Check sheet for the modelled part. Datum: model origin and axes. Units: mm. A direction names the side the tool comes from. Coordinates: 2 decimals unless noted, no trailing zeros. Order: outer loops, then holes, each group sorted by start corner. A loop starts at its lowest first (then second) coordinate and runs counter-clockwise, first axis right, second up.
1. Cross-section at D-D (y = -27). Enter the section's corners in (x, z).
2. Draft check along X on faces 4 (the flat face through (-12, -50.8, 24)), 5 (the flat face through (8.028, -13, 41)), 6 (the flat face through (31.87, -12.52, -27.67)). Enter one of: released by +X, released by -X, zero draft, split by the parting line, or undercut.
3. Gauge pin test, flat ends, axial feed: pin 1 Ø10 at (x, y) = (-31.5, -21.5) entering from -Z; pin 2 Ø22.5 at (x, z) = (-5.5, -4.5) entering from -Y; pin 3 Ø4 at (y, z) = (-7.5, 43) entering from +X. Record the tip position at first contact, or that the pin passes through.
4. Cross-section at B-B (z = 0). Enter the section's corners in (x, y).
5. Cross-section at C-C (x = -39.5). Enter the section's corners in (y, z), then the cut area to 3 significant figures.
6. Set-up check for faces 1 (the flat face through (-8.028, -13, 42)), 2 (the flat face through (11, -25.4, -11)), 3 (the cylindrical face through (-45.124, -12.878, -26.684)): record each of +Z, -Z, +X, -X, +Y, -Y from which the full face is reachable in a straight line by a thin tool's end or side.
7. Cross-section at A-A (x = 0). Enter the section's corners in (y, z), then the cut area to 3 significant figures.
8. Thickness scan on line 1 (Z direction, x = 0, y = -20); line 2 (Z direction, x = 0, y = -10); line 3 (Z direction, x = 0, y = -37.5). Record the ranges inside material, lowest first.
```python
from build123d import *

# Parameters (mm, degrees)
F1_DEPTH  = 25.4
F2_R      = 4.203451
F3_DEPTH  = 25.401
F4_R      = 6.269699
F4_R_2    = 4.203451
F6_DEPTH  = 12.7
F7_R      = 9.142081
F8_DEPTH  = 25.401
F9_R      = 13.925159
F10_DEPTH = 12.7
F11_R     = 31.560362
F11_R_2   = 26.120651
F12_DEPTH = 25.4


with BuildPart() as f1:
    # F0 (on Front) → F1 (new body)
    with BuildSketch(Plane.XZ):
        with BuildLine():
            Line((-8.028061, 48.252545), (-8.028061, 34.79823))
            ThreePointArc((-8.028061, 34.79823), (-30.927737, 17.856137), (-34.150182, -10.44661))
            ThreePointArc((-34.150182, -10.44661), (-30.927737, -17.856137), (-26.122121, -24.35162))
            ThreePointArc((-26.122121, -24.35162), (0, -35.712275), (26.122121, -24.35162))
            ThreePointArc((26.122121, -24.35162), (30.927737, -17.856137), (34.150182, -10.44661))
            ThreePointArc((34.150182, -10.44661), (30.927737, 17.856137), (8.028061, 34.79823))
            Line((8.028061, 34.79823), (8.028061, 48.252545))
            ThreePointArc((8.028061, 48.252545), (0, 56.280606), (-8.028061, 48.252545))
        make_face()
        with BuildLine():
            ThreePointArc((-26.122121, -24.35162), (-30.927737, -17.856137), (-34.150182, -10.44661))
            Line((-34.150182, -10.44661), (-45.801961, -17.173768))
            ThreePointArc((-45.801961, -17.173768), (-48.740435, -28.140303), (-37.773899, -31.078778))
            Line((-37.773899, -31.078778), (-26.122121, -24.35162))
        make_face()
        with BuildLine():
            ThreePointArc((34.150182, -10.44661), (30.927737, -17.856137), (26.122121, -24.35162))
            Line((26.122121, -24.35162), (37.773899, -31.078778))
            ThreePointArc((37.773899, -31.078778), (48.740435, -28.140303), (45.801961, -17.173768))
            Line((45.801961, -17.173768), (34.150182, -10.44661))
        make_face()
    extrude(amount=F1_DEPTH)

    # F2 (on face) → F3 (cut, through all)
    with BuildSketch(Plane.XZ.offset(25.4)):
        with Locations((0, 48.252545)):
            Circle(F2_R)
        with Locations((-41.78793, -24.126273)):
            Circle(F2_R)
        with Locations((41.78793, -24.126273)):
            Circle(F2_R)
    extrude(amount=-F3_DEPTH, mode=Mode.SUBTRACT)

    # F4 (on face) → F6 (cut)
    with BuildSketch(Plane.XZ.offset(25.4)):
        with Locations((0, 48.252545)):
            Circle(F4_R)
        with Locations((0, 48.252545)):
            Circle(F4_R_2, mode=Mode.SUBTRACT)
    extrude(amount=-F6_DEPTH, mode=Mode.SUBTRACT)

    # F7 (on face) → F8 (cut, through all)
    with BuildSketch(Plane.XZ.offset(25.4)):
        Circle(F7_R)
    extrude(amount=-F8_DEPTH, mode=Mode.SUBTRACT)

    # F9 (on face) → F10 (cut)
    with BuildSketch(Plane.XZ.offset(25.4)):
        Circle(F9_R)
    extrude(amount=-F10_DEPTH, mode=Mode.SUBTRACT)

    # F11 (on face) → F12 (join)
    with BuildSketch(Plane.XZ.offset(25.4)):
        Circle(F11_R)
        Circle(F11_R_2, mode=Mode.SUBTRACT)
    extrude(amount=F12_DEPTH)


solid = f1.part
```
Data:
1. outline: circle Ø63.12 at (0, 0); hole circle Ø52.24 at (0, 0)
2. face 4: zero draft
2. face 5: released by +X
2. face 6: undercut
3. pin 1: stops at z = -30.34
3. pin 2: stops at y = -25.4
3. pin 3: stops at x = 8.03
4. outline: (-35.71, -25.4) - (-31.56, -25.4) - (-31.56, -50.8) - (-26.12, -50.8) - (-26.12, -25.4) - (-13.93, -25.4) - (-13.93, -12.7) - (-9.14, -12.7) - (-9.14, 0) - (-35.71, 0) - close; (9.14, -12.7) - (13.93, -12.7) - (13.93, -25.4) - (26.12, -25.4) - (26.12, -50.8) - (31.56, -50.8) - (31.56, -25.4) - (35.71, -25.4) - (35.71, 0) - (9.14, 0) - close
5. outline: (-25.4, -31.82) - (0, -31.82) - (0, -27.65) - (-25.4, -27.65) - close; (-25.4, -20.6) - (0, -20.6) - (0, -13.54) - (-25.4, -13.54) - close
5. area: 285 mm2
6. face 1: +Z, -X, +Y, -Y
6. face 2: -Y
6. face 3: +Y, -Y
7. outline: (-50.8, -31.56) - (-25.4, -31.56) - (-25.4, -35.71) - (0, -35.71) - (0, -9.14) - (-12.7, -9.14) - (-12.7, -13.93) - (-25.4, -13.93) - (-25.4, -26.12) - (-50.8, -26.12) - close; (-50.8, 26.12) - (-25.4, 26.12) - (-25.4, 13.93) - (-12.7, 13.93) - (-12.7, 9.14) - (0, 9.14) - (0, 44.05) - (-12.7, 44.05) - (-12.7, 41.98) - (-25.4, 41.98) - (-25.4, 31.56) - (-50.8, 31.56) - close; (-25.4, 54.52) - (-12.7, 54.52) - (-12.7, 52.46) - (0, 52.46) - (0, 56.28) - (-25.4, 56.28) - close
7. area: 1,760 mm2
8. line 1: z = -35.71 to -13.93, 13.93 to 41.98, 54.52 to 56.28
8. line 2: z = -35.71 to -9.14, 9.14 to 44.05, 52.46 to 56.28
8. line 3: z = -31.56 to -26.12, 26.12 to 31.56
